Input: part model. Units: mm. Frame: model coordinates. Give positions to 0.01 mm unless a question says otherwise; leave off trailing zeros. Loops run counter-clockwise (first coordinate to the right, second up) from the corner with the lowest first, then second, coordinate; pieces in that order, holes last. Notation, with made-up numbers: (82, 73) -> (103, 73) arc R22 ccw to (103, 97) -> close; hole circle Ø2 at (83, 25.5). An arc over 180 degrees is marked (long way). Answer in a Markdown table with one row per item. Add a question column.
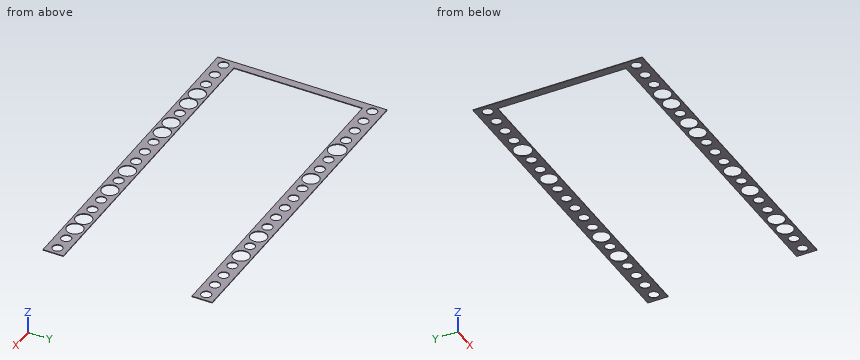
```python
from build123d import *

# Parameters (mm, degrees)
F0_R     = 0.7326874882
F0_R_2   = 1.3
F0_R_3   = 1.2
F0_W     = 1.1555750221
F0_H     = 19
F1_DEPTH = 0.1


# Not quite as in the source:
# - a feature names something its author has since deleted; it is built from what else it names


with BuildPart() as f1:
    # F0 (on Top) → F1 (new body)
    with BuildSketch(Plane.XY):
        Polygon((24.25, 14.5), (-24.25, 14.5), (-24.25, 11.5), (-23.0944249779, 11.5), (-1.1800766224, 11.5), (1.0609005112, 11.5), (24.25, 11.5), align=None)
        with Locations((-23.0375, 12.9655366763)):
            Circle(F0_R, mode=Mode.SUBTRACT)
        with Locations((-20.6125, 12.9655366763)):
            Circle(F0_R, mode=Mode.SUBTRACT)
        with Locations((-18.1875, 12.9655366763)):
            Circle(F0_R, mode=Mode.SUBTRACT)
        with Locations((-15.7625, 12.9655366763)):
            Circle(F0_R, mode=Mode.SUBTRACT)
        with Locations((-13.3375, 12.9655366763)):
            Circle(F0_R_2, mode=Mode.SUBTRACT)
        with Locations((-10.9125, 12.9655366763)):
            Circle(F0_R, mode=Mode.SUBTRACT)
        with Locations((-8.4875, 12.9655366763)):
            Circle(F0_R, mode=Mode.SUBTRACT)
        with Locations((-6.0625, 12.9655366763)):
            Circle(F0_R_3, mode=Mode.SUBTRACT)
        with Locations((-3.6375, 12.9655366763)):
            Circle(F0_R, mode=Mode.SUBTRACT)
        with Locations((-1.2125, 12.9655366763)):
            Circle(F0_R, mode=Mode.SUBTRACT)
        with Locations((1.2125, 12.9655366763)):
            Circle(F0_R, mode=Mode.SUBTRACT)
        with Locations((3.6375, 12.9655366763)):
            Circle(F0_R, mode=Mode.SUBTRACT)
        with Locations((6.0625, 12.9655366763)):
            Circle(F0_R, mode=Mode.SUBTRACT)
        with Locations((8.4875, 12.9655366763)):
            Circle(F0_R_3, mode=Mode.SUBTRACT)
        with Locations((10.9125, 12.9655366763)):
            Circle(F0_R, mode=Mode.SUBTRACT)
        with Locations((13.3375, 12.9655366763)):
            Circle(F0_R_3, mode=Mode.SUBTRACT)
        with Locations((15.7625, 12.9655366763)):
            Circle(F0_R, mode=Mode.SUBTRACT)
        with Locations((18.1875, 12.9655366763)):
            Circle(F0_R, mode=Mode.SUBTRACT)
        with Locations((20.6125, 12.9655366763)):
            Circle(F0_R, mode=Mode.SUBTRACT)
        with Locations((23.0375, 12.9655366763)):
            Circle(F0_R, mode=Mode.SUBTRACT)
        Polygon((-23.0944249779, -7.5), (-24.25, -7.5), (-24.25, -10.5), (24.25, -10.5), (24.25, -7.5), (1.0609005112, -7.5), (-1.1800766224, -7.5), align=None)
        with Locations((-23.0375, -9.0053491294)):
            Circle(F0_R, mode=Mode.SUBTRACT)
        with Locations((-20.6125, -9.0053491294)):
            Circle(F0_R, mode=Mode.SUBTRACT)
        with Locations((-18.1875, -9.0053491294)):
            Circle(F0_R, mode=Mode.SUBTRACT)
        with Locations((-15.7625, -9.0053491294)):
            Circle(F0_R_3, mode=Mode.SUBTRACT)
        with Locations((-13.3375, -9.0053491294)):
            Circle(F0_R_3, mode=Mode.SUBTRACT)
        with Locations((-10.9125, -9.0053491294)):
            Circle(F0_R, mode=Mode.SUBTRACT)
        with Locations((-8.4875, -9.0053491294)):
            Circle(F0_R_3, mode=Mode.SUBTRACT)
        with Locations((-6.0625, -9.0053491294)):
            Circle(F0_R_3, mode=Mode.SUBTRACT)
        with Locations((-3.6375, -9.0053491294)):
            Circle(F0_R, mode=Mode.SUBTRACT)
        with Locations((-1.2125, -9.0053491294)):
            Circle(F0_R, mode=Mode.SUBTRACT)
        with Locations((1.2125, -9.0053491294)):
            Circle(F0_R, mode=Mode.SUBTRACT)
        with Locations((3.6375, -9.0053491294)):
            Circle(F0_R_3, mode=Mode.SUBTRACT)
        with Locations((6.0625, -9.0053491294)):
            Circle(F0_R, mode=Mode.SUBTRACT)
        with Locations((8.4875, -9.0053491294)):
            Circle(F0_R_3, mode=Mode.SUBTRACT)
        with Locations((10.9125, -9.0053491294)):
            Circle(F0_R, mode=Mode.SUBTRACT)
        with Locations((13.3375, -9.0053491294)):
            Circle(F0_R, mode=Mode.SUBTRACT)
        with Locations((15.7625, -9.0053491294)):
            Circle(F0_R_3, mode=Mode.SUBTRACT)
        with Locations((18.1875, -9.0053491294)):
            Circle(F0_R_3, mode=Mode.SUBTRACT)
        with Locations((20.6125, -9.0053491294)):
            Circle(F0_R, mode=Mode.SUBTRACT)
        with Locations((23.0375, -9.0053491294)):
            Circle(F0_R, mode=Mode.SUBTRACT)
        with Locations((-23.6722124889, 2)):
            Rectangle(F0_W, F0_H)
    extrude(amount=F1_DEPTH)


solid = f1.part
```
1) Section B-B on y = -7. Output: boundary loops of the cut face in (x, z), and give its area (3 significant figures).
2) Material intervals for line 1 along Y through (x, z) = (13.5, 0.05); line 2 along Y through (x, z) = (13, 0.05); line 3 along X through (y, z) = (5.25, 0.05), sorted ascending.
3) Section A-A on x = -11. Output: boundary loops of the cut face in (y, z), and give its area (3 significant figures).
4) Section C-C on z = 0.05. State how many separate pieces and enclosed holes the cut face has, and give its area (3 significant figures).
Working result:
| question | item | result |
|---|---|---|
| 1 | outline | (-24.25, 0) -> (-23.09, 0) -> (-23.09, 0.1) -> (-24.25, 0.1) -> close |
| 1 | area | 0.116 mm2 |
| 2 | line 1 | y = -10.5 to -9.72, -8.29 to -7.5, 11.5 to 11.78, 14.15 to 14.5 |
| 2 | line 2 | y = -10.5 to -9.66, -8.36 to -7.5, 11.5 to 11.81, 14.12 to 14.5 |
| 2 | line 3 | x = -24.25 to -23.09 |
| 3 | outline | (-10.5, 0) -> (-9.73, 0) -> (-9.73, 0.1) -> (-10.5, 0.1) -> close; (-8.28, 0) -> (-7.5, 0) -> (-7.5, 0.1) -> (-8.28, 0.1) -> close; (11.5, 0) -> (12.24, 0) -> (12.24, 0.1) -> (11.5, 0.1) -> close; (13.69, 0) -> (14.5, 0) -> (14.5, 0.1) -> (13.69, 0.1) -> close |
| 3 | area | 0.309 mm2 |
| 4 | separate pieces | 1 |
| 4 | enclosed holes | 40 |
| 4 | area | 211 mm2 |
